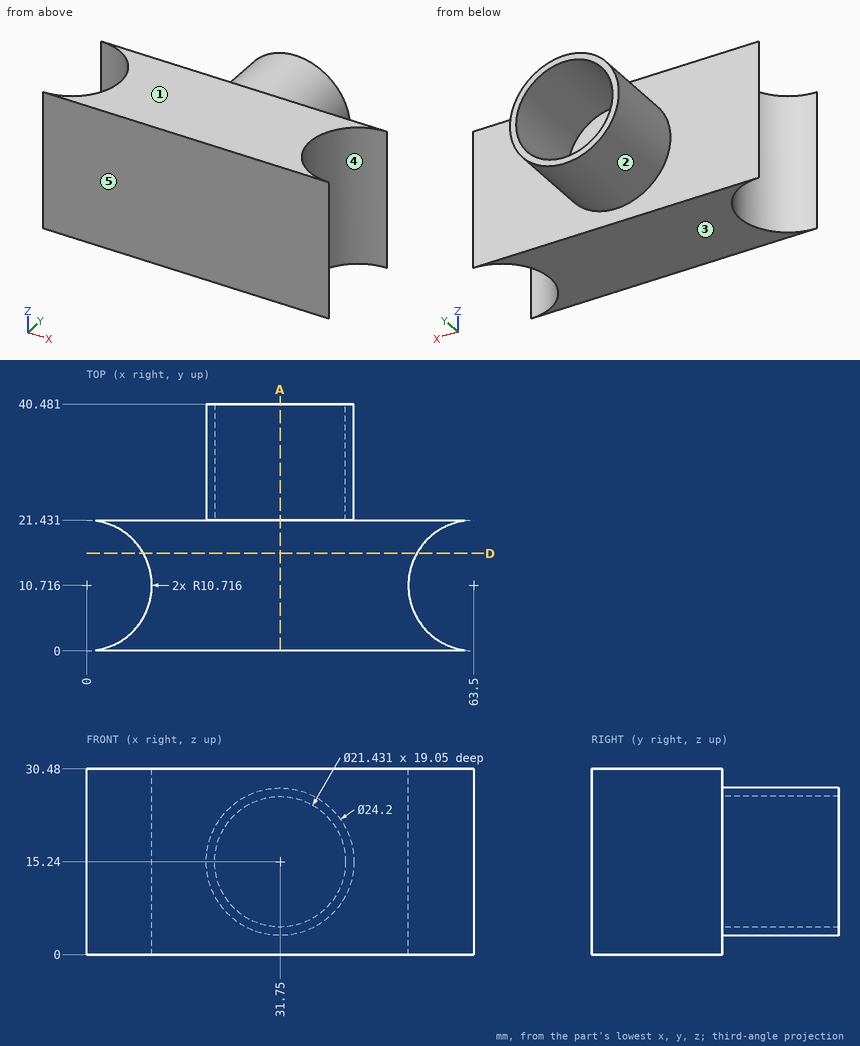
Geometry check sheet. Reference: drawing and pictorial views, mm from the part's lowest x, y, z. A direction names the side the tool comes from. Give positions to 0.01 mm unless a question says otherwise; leave off trailing zeros. Write each loop counter-clockwise with the first axis right and the second up, starting at its lowest first coordinate (ties: lowest second). Pieces come first, ordered by that corner, then holes.
Item 1: Gauge pin test, flat ends, axial feed: pin 1 (10 mm diameter, centred on x = 23.5, z = 20.5, fed in from +Y); pin 2 (1.5 mm diameter, centred on y = 8.5, z = 20.5, fed in from +X); pin 3 (5 mm diameter, centred on x = 23, y = 30, fed in from -Z); pin 4 (8 mm diameter, centred on y = 31.5, z = 9, fed in from +X). Record the tip position at first contact, or that the pin passes through.
Item 2: Cross-section at D-D (y = 16). Enter the section's corners in (x, z).
Item 3: Scan lines: L1, parallel to Z at x = 31.75, y = 30 (1 decimal); L2, parallel to Z at x = 31, y = 30; L3, parallel to Y at x = 48, z = 18. Record each from-to range of solid material in increasing order.
Item 4: Draft check along Y on the marked faces 3, 4 and 5. Enter one of: released by +Y, released by -Y, zero draft, split by the parting line, or undercut.
Item 5: Cross-section at A-A (x = 31.75). Enter the section's corners in (y, z) (1 decimal).
Item 6: Access from +Z, -Z, +X, -X, +Y, -Y to the whole of each face (thin tool, end or side, straight path). Record for the marked faces 1 and 2.
Report:
1. pin 1: stops at y = 40.48
1. pin 2: stops at x = 53.2
1. pin 3: stops at z = 4.88
1. pin 4: stops at x = 43.64
2. outline: (9.32, 0) - (54.18, 0) - (54.18, 30.48) - (9.32, 30.48) - close
3. L1: z = 3.1 to 4.5, 26 to 27.3
3. L2: z = 3.16 to 4.55, 25.93 to 27.32
3. L3: y = 0 to 21.43
4. face 3: zero draft
4. face 4: undercut
4. face 5: released by -Y
5. outline: (0, 0) - (21.4, 0) - (21.4, 3.1) - (40.5, 3.1) - (40.5, 4.5) - (21.4, 4.5) - (21.4, 26) - (40.5, 26) - (40.5, 27.3) - (21.4, 27.3) - (21.4, 30.5) - (0, 30.5) - close
6. face 1: +Z, +X, -X, +Y, -Y
6. face 2: +Y
